The figure shows three views and two pictorial views of one solid part (mm, origin at its lowest corner). Answer the questions. Give positions to 0.01 mm unless a question says otherwise; leave off trailing zeros. Order: outer loops, then holes, each group sorted by start corner. A loop starts at its lowest first (then second) coordinate and runs counter-clockwise, first axis right, second up. Notation, with made-up numbers: M -2.5,67 L 8.5,67 A32 ccw 8.5,95 Z; hole C 40,-31.75 d2. An arc over 180 degrees is marked long. One line per item, written item: value. Start each with the question number.
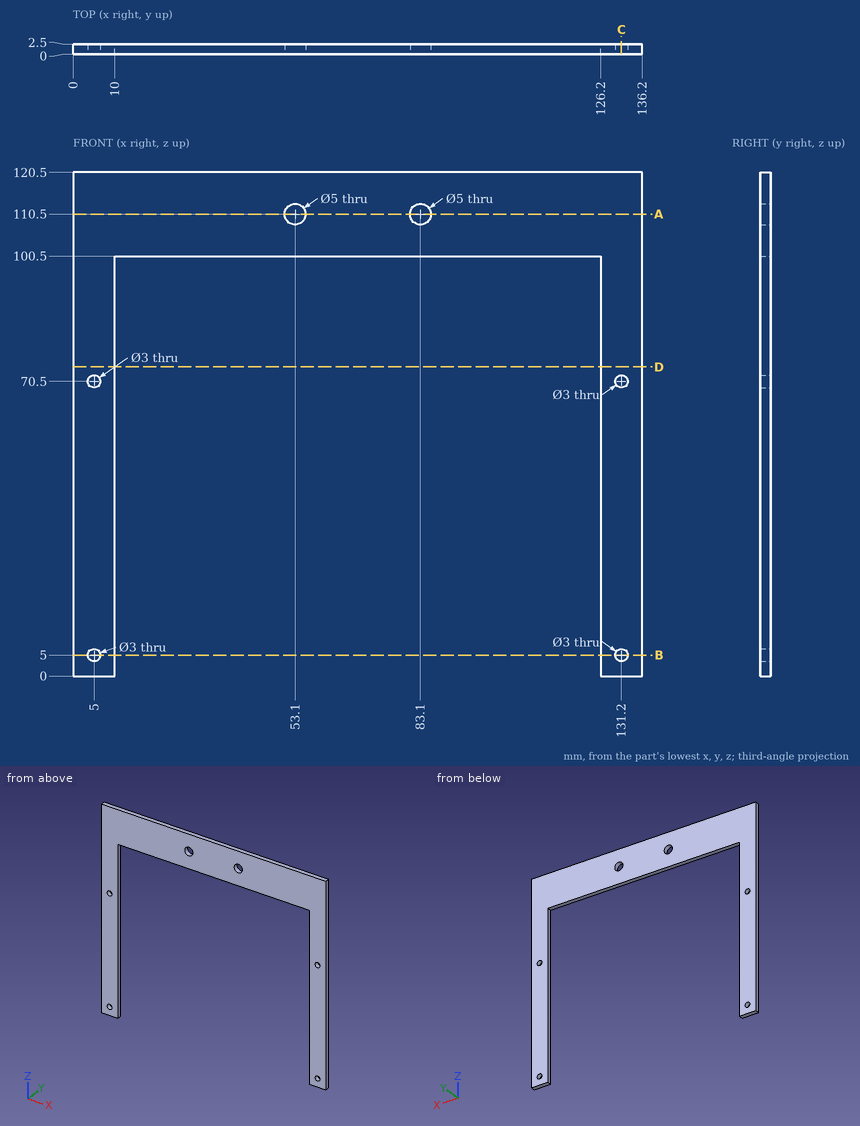
Q1. Find section B-B, the plane z = 5. Give the vertices of the cut face in (x, y), then the cut area to 3 significant figures.
Q2. Find section C-C, the plane x = 131.2. Give the vertices of the cut face in (y, z).
Q3. Find section A-A, the plane z = 110.5. Give the vertices of the cut face in (x, y).
Q4. Consider probe 1 along X at (y, z) = (0.55, 70.5); probe 2 along X at (y, z) = (1.85, 43.5); probe 3 along X at (y, z) = (1.5, 112.5). Determine where each line is inside the solid, lowest interval first.
Q5. Each of these flat-tipped pins is pushed along its axis until it touches: pin 1 (1.2 mm diameter, centred on x = 91.5, y = 1, fed in from -Z); pin 2 (5 mm diameter, centred on x = 131.2, z = 5, fed in from -Y); pin 3 (2.5 mm diameter, centred on x = 5, z = 5, fed in from -Y). Where does it stop, or does it pass through?
Q6. Find section D-D, the plane z = 74. Give the vertices of the cut face in (x, y).
Evaluation:
1. outline: M 0,0 L 3.5,0 L 3.5,2.5 L 0,2.5 Z; M 6.5,0 L 10,0 L 10,2.5 L 6.5,2.5 Z; M 126.2,0 L 129.7,0 L 129.7,2.5 L 126.2,2.5 Z; M 132.7,0 L 136.2,0 L 136.2,2.5 L 132.7,2.5 Z
1. area: 35.0 mm2
2. outline: M 0,0 L 2.5,0 L 2.5,3.5 L 0,3.5 Z; M 0,6.5 L 2.5,6.5 L 2.5,69 L 0,69 Z; M 0,72 L 2.5,72 L 2.5,120.5 L 0,120.5 Z
3. outline: M 0,0 L 50.6,0 L 50.6,2.5 L 0,2.5 Z; M 55.6,0 L 80.6,0 L 80.6,2.5 L 55.6,2.5 Z; M 85.6,0 L 136.2,0 L 136.2,2.5 L 85.6,2.5 Z
4. probe 1: 0 to 3.5, 6.5 to 10, 126.2 to 129.7, 132.7 to 136.2
4. probe 2: 0 to 10, 126.2 to 136.2
4. probe 3: 0 to 51.6, 54.6 to 81.6, 84.6 to 136.2
5. pin 1: z = 100.5
5. pin 2: y = 0
5. pin 3: through
6. outline: M 0,0 L 10,0 L 10,2.5 L 0,2.5 Z; M 126.2,0 L 136.2,0 L 136.2,2.5 L 126.2,2.5 Z
